Here's how the part is built. I have some questions about the finished solid (model axes, mm). A direction names the side the tool comes from. Round coordinates to 2 decimals unless told otherwise and drop trailing zeros. Write each loop counter-clockwise with the first axis right and the second up, starting at its lowest first coordinate (ties: lowest second). Pieces come first, ordered by that corner, then holes. Notation, with made-up numbers: (61.25, 6) - (82.25, 6) arc R30 cw to (82.25, 39) - close; hole circle Ø2 at (41.5, -18). An arc over 180 degrees is marked (long way). One line per question, with ' | ' between items. Start each with the question number.
(1) Thinking about a two-plate mould opening in X: for faces 1 (the flat face through (5, 0, 0)), 2 (the cylindrical face through (0, -10, 13)), 3 (the cylindrical face through (-14.985, 0.66, 12.972)), which applies, pulls with the +X half, pulls with the -X half, needs draft (parallel to the pull), parting line crosses it, or undercut?
(2) If I drill on L1, parallel to Y at x = 0, z = 6.05; L2, parallel to Y at x = 0, z = 12.7; L3, parallel to Y at x = 0, z = 2, over which ranges is the centre line in solid material (lowest first)?
(3) Will these pins go through, and if not, where does the flat tip stop? pin 1 (3 mm diameter, centred on y = 2, z = 8, fed in from +X); pin 2 (5 mm diameter, centred on y = -9.5, z = 7, fed in from +X); pin 3 (2.5 mm diameter, centred on x = 0, y = 11, fed in from +Z); pin 4 (0.7 mm diameter, centred on x = -8, y = 0.5, fed in from -Z).
(4) Imagine slicing it at A-A (z = 9.5). Write out the boundary of the cut face in (x, y).
(5) For faces 4 (the cylindrical face through (0.65, 8.76, 3.45)), 5 (the flat face through (0, -3, 15)), 6 (the flat face through (3, -10, 11)), 7 (the cylindrical face through (0, 10, 13)), which set-ups out of +Z, -Z, +X, -X, +Y, -Y let a thin tool reach every point of the face, with its end or its side?
(6) Imagine slicing it at D-D (x = -10.75). Write out the boundary of the cut face in (y, z).
(7) Imagine slicing it at B-B (z = 2.5). Write out the boundary of the cut face in (x, y), plus the area to 3 significant figures.
(8) Imagine slicing it at C-C (y = -11). Write out the boundary of the cut face in (x, z), plus the area to 3 significant figures.
from build123d import *

# Parameters (mm, degrees)
SKETCH1_R           = 15
SKETCH1_R_2         = 1.2
SKETCH1_W           = 9.3
SKETCH1_H           = 9.3
BOSS_EXTRUDE1_DEPTH = 7
SKETCH2_R           = 10
SKETCH2_R_2         = 1.5
SKETCH2_W           = 1.35
SKETCH2_H           = 9.3
BOSS_EXTRUDE2_DEPTH = 4
SKETCH3_R           = 15
SKETCH3_R_2         = 1.5
BOSS_EXTRUDE3_DEPTH = 4
SKETCH4_R           = 15
SKETCH4_R_2         = 12
CUT_EXTRUDE1_DEPTH  = 4
SKETCH5_R           = 1
CUT_EXTRUDE2_DEPTH  = 3
SKETCH6_R           = 1
CUT_EXTRUDE5_DEPTH  = 5


with BuildPart() as part:
    # Sketch1 → Boss-Extrude1 (new body)
    with BuildSketch(Plane.XY):
        Circle(SKETCH1_R)
        with Locations((0, 7.75)):
            Circle(SKETCH1_R_2, mode=Mode.SUBTRACT)
        with Locations((7.75, 0)):
            Circle(SKETCH1_R_2, mode=Mode.SUBTRACT)
        with Locations((0, -7.75)):
            Circle(SKETCH1_R_2, mode=Mode.SUBTRACT)
        with Locations((-7.75, 0)):
            Circle(SKETCH1_R_2, mode=Mode.SUBTRACT)
        Rectangle(SKETCH1_W, SKETCH1_H, mode=Mode.SUBTRACT)
    extrude(amount=BOSS_EXTRUDE1_DEPTH)

    # Sketch2 → Boss-Extrude2 (add)
    with BuildSketch(Plane.XY.offset(7)):
        Circle(SKETCH2_R)
        Circle(SKETCH2_R_2, mode=Mode.SUBTRACT)
        with Locations((-3.975, 0)):
            Rectangle(SKETCH2_W, SKETCH2_H, mode=Mode.SUBTRACT)
        with Locations((3.975, 0)):
            Rectangle(SKETCH2_W, SKETCH2_H, mode=Mode.SUBTRACT)
    extrude(amount=BOSS_EXTRUDE2_DEPTH)

    # Sketch3 → Boss-Extrude3 (add)
    with BuildSketch(Plane.XY.offset(11)):
        Circle(SKETCH3_R)
        Circle(SKETCH3_R_2, mode=Mode.SUBTRACT)
    extrude(amount=BOSS_EXTRUDE3_DEPTH)

    # Sketch4 → Cut-Extrude1 (cut)
    with BuildSketch(Plane(origin=(0, 0, 0), x_dir=(-1, 0, 0), z_dir=(0, 0, -1))):
        Circle(SKETCH4_R)
        Circle(SKETCH4_R_2, mode=Mode.SUBTRACT)
    extrude(amount=-CUT_EXTRUDE1_DEPTH, mode=Mode.SUBTRACT)

    # Sketch5 → Cut-Extrude2 (cut)
    with BuildSketch(Plane(origin=(0, 0, 4), x_dir=(-1, 0, 0), z_dir=(0, 0, -1))):
        with Locations((0, 13)):
            Circle(SKETCH5_R)
        with Locations((0, -13)):
            Circle(SKETCH5_R)
    extrude(amount=-CUT_EXTRUDE2_DEPTH, mode=Mode.SUBTRACT)

    # Sketch6 → Cut-Extrude5 (cut, through all)
    with BuildSketch(Plane(origin=(0, 0, 11), x_dir=(-1, 0, 0), z_dir=(0, 0, -1))):
        with Locations((0, 11)):
            Circle(SKETCH6_R)
        with Locations((0, -11)):
            Circle(SKETCH6_R)
    extrude(amount=-CUT_EXTRUDE5_DEPTH, mode=Mode.SUBTRACT)


solid = part.part
Check sheet entries:
1) face 1: needs draft | face 2: undercut | face 3: parting line crosses it
2) L1: -15 to -14, -12 to -8.95, -6.55 to -4.65, 4.65 to 6.55, 8.95 to 12, 14 to 15 | L2: -15 to -12, -10 to -1.5, 1.5 to 10, 12 to 15 | L3: -12 to -8.95, -6.55 to -4.65, 4.65 to 6.55, 8.95 to 12
3) pin 1: x = 14.97 | pin 2: x = 13.27 | pin 3: z = 15 | pin 4: z = 7
4) outline: circle Ø20 at (0, 0); hole (-4.65, -4.65) - (-3.3, -4.65) - (-3.3, 4.65) - (-4.65, 4.65) - close; hole circle Ø3 at (0, 0); hole (3.3, -4.65) - (4.65, -4.65) - (4.65, 4.65) - (3.3, 4.65) - close
5) face 4: -Z | face 5: +Z, +X, -X, +Y, -Y | face 6: none | face 7: +Z
6) outline: (-10.46, 4) - (-5.33, 4) - (-5.33, 0) - (5.33, 0) - (5.33, 4) - (10.46, 4) - (10.46, 7) - (-10.46, 7) - close; (-10.46, 11) - (10.46, 11) - (10.46, 15) - (-10.46, 15) - close
7) outline: circle Ø24 at (0, 0); hole circle Ø2.4 at (-7.75, 0); hole (-4.65, -4.65) - (4.65, -4.65) - (4.65, 4.65) - (-4.65, 4.65) - close; hole circle Ø2.4 at (0, -7.75); hole circle Ø2.4 at (0, 7.75); hole circle Ø2.4 at (7.75, 0) | area: 348 mm^2
8) outline: (-10.2, 4) - (-4.8, 4) - (-4.8, 0) - (4.8, 0) - (4.8, 4) - (10.2, 4) - (10.2, 7) - (-10.2, 7) - close; (-10.2, 11) - (-1, 11) - (-1, 15) - (-10.2, 15) - close; (1, 11) - (10.2, 11) - (10.2, 15) - (1, 15) - close | area: 173 mm^2
